Print and shaded views of the part. All mm, measured from the part's lowest x, y and z. Round coordinates to 2 decimals unless told otherwise and drop trailing zeros. Order: outer loops, then holes, each group sorted by start corner. A loop starts at its lowest first (then second) coordinate and runs counter-clockwise, first axis right, second up. Notation, with made-up numbers: (-15.5, 30.5) - (-6.5, 30.5) arc R30 ccw to (-6.5, 58.5) - close; hole circle Ø7 at (-3, 79.5). An arc over 180 degrees is marked (long way). Write item = value, one per line.
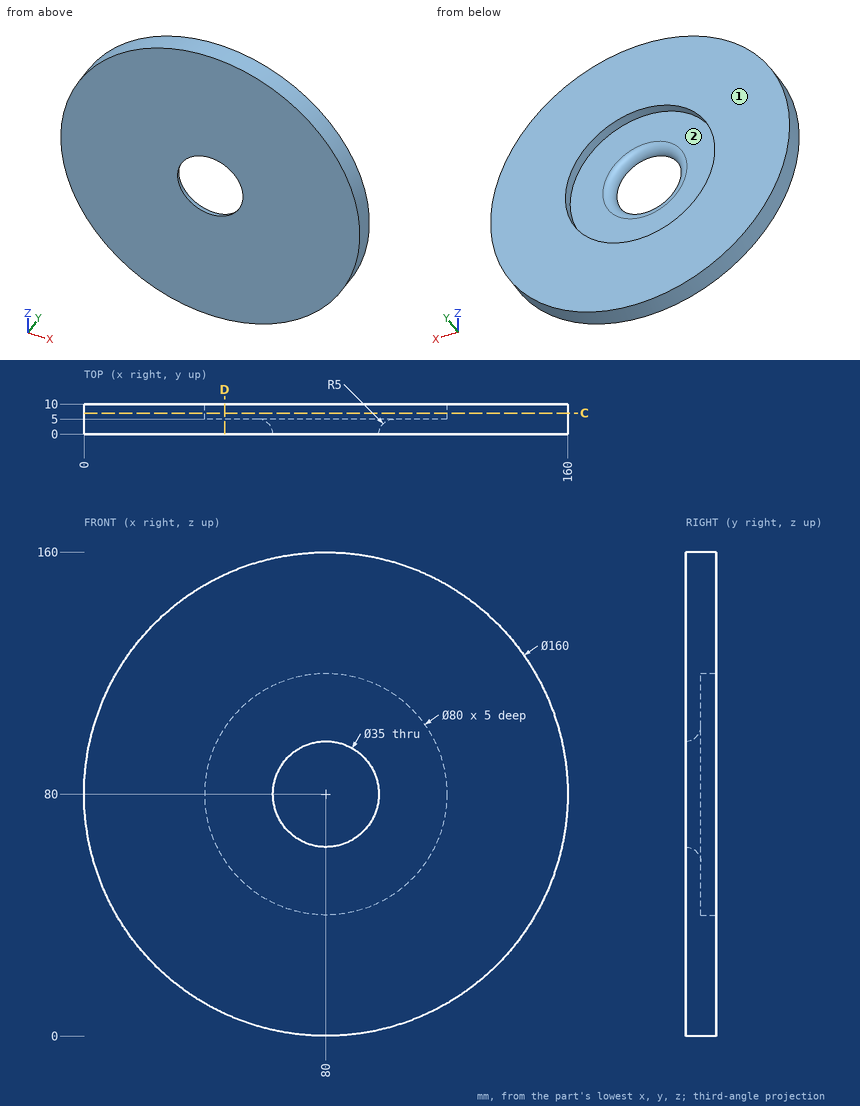
(1) Probe line 1 along X through (y, z) = (8.25, 81); line 2 along Z through (x, y) = (80, 8.2); line 3 along Z through (x, y) = (55, 8.5) (1 decimal). List the from-to ranges inside material, lowest first.
Solved:
line_1 = 0.01 to 40.01, 119.99 to 159.99
line_2 = 0 to 40, 120 to 160
line_3 = 4 to 48.8, 111.2 to 156
(2) Band-saw the part on D-D on x = 46.5. List the corners of the cut face in (y, z).
Solved:
outline = (0, 7.35) - (10, 7.35) - (10, 58.14) - (5, 58.14) - (5, 101.86) - (10, 101.86) - (10, 152.65) - (0, 152.65) - close
(3) Pull direction X, two halves, no side cores. Call the marked faces 1 and 2: released by +X, released by -X, zero draft, split by the parting line, or undercut.
Solved:
face_1 = zero draft
face_2 = undercut
(4) Drop flat-ended pins along their axis: pin 1 (5 mm diameter, centred on y = 9, z = 45, fed in from -X); pin 2 (3 mm diameter, centred on y = 6.5, z = 27.5, fed in from +X) (1 decimal); pin 3 (2 mm diameter, centred on x = 95, y = 3.5, fed in from +Z) (1 decimal). Give the stop position or say it passes through.
Solved:
pin_1 = 6.9
pin_2 = 141.6
pin_3 = 158.8
(5) Band-saw the part on C-C on y = 7. List the corners of the cut face in (x, z).
Solved:
outline = circle Ø160 at (80, 80); hole circle Ø80 at (80, 80)
